Answer from the drawing. Dimensions are ordinates in mm from the lowest x, y and z of the part. A direction names the side the tool comes from. Coordinates: 2 decimals unless noted, no trailing zeros. Order: outer loops, then holes, each group sorted by start corner. A loop starts at its lowest first (then second) coordinate and runs counter-clockwise, first axis right, second up. Notation, with made-up numbers: (-11.5, 40.5) - (14.5, 40.5) arc R11 ccw to (14.5, 46.5) - close; hole circle Ø5 at (3, 69). An arc over 180 degrees is marked (long way). Answer as a JSON object with one key per item and string values. Group by question number.
1) Section C-C (y = 21) is taken. Give the vertices of the cut face in (x, z).
2) Section B-B (z = 1.95) is taken. Give the vertices of the cut face in (x, y).
3) Each of these flat-tipped pins is pushed along its axis until it touches: P1, Ø1, axis at x = 1, y = 21.5, coming from the -Z side; P2, Ø0.8, axis at x = 2.5, z = 3, coming from the +Y side. Where does it stop, or does it pass through?
4) The mould has two halves that part along X. Classify the marked faces 1, 2 and 3: released by +X, released by -X, zero draft, split by the parting line, or undercut.
5) Find the intervals of material crossed by line 1 along Z through (x, y) = (2.7, 9.5); line 2 along Y through (x, z) = (1.35, 4.45); line 3 along Y through (x, z) = (3.1, 2.4), in increasing order.
6) A tool of negligible diameter and unlimited length cuts with its end or side. For the marked faces 4 and 5, from which of +Z, -Z, +X, -X, +Y, -Y can it reach the whole face along a straight path? Write none if from no direction.
7) Section D-D (x = 0.5) is taken. Give the vertices of the cut face in (y, z).
8) Section A-A (x = 2.75) is taken. Give the vertices of the cut face in (y, z).
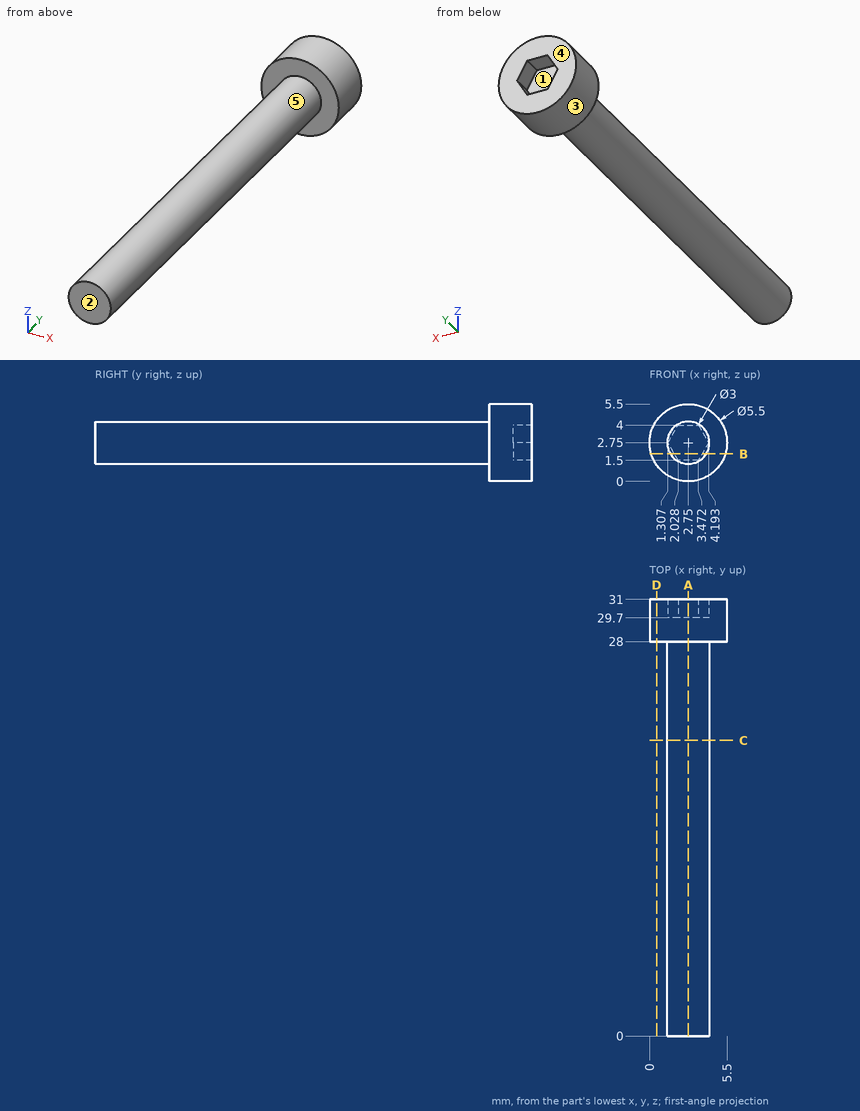
Report:
{
 "1": {"outline": "circle Ø3 at (2.75, 2.75)"},
 "2": {"outline": "(0.12, 28) - (1.48, 28) - (1.48, 0) - (4.02, 0) - (4.02, 28) - (5.38, 28) - (5.38, 31) - (3.73, 31) - (3.73, 29.7) - (1.77, 29.7) - (1.77, 31) - (0.12, 31) - close"},
 "3": {"P1": "stops at z = 1.92", "P2": "stops at y = 29.7"},
 "4": {"face 1": "undercut", "face 2": "zero draft", "face 3": "split by the parting line"},
 "5": {"line 1": "z = 1.25 to 4.25", "line 2": "y = 28 to 31", "line 3": "y = 0 to 29.7"},
 "6": {"face 4": "+Z, -Z, +X, -X, +Y", "face 5": "-Y"},
 "7": {"outline": "(28, 1.17) - (31, 1.17) - (31, 4.33) - (28, 4.33) - close"},
 "8": {"outline": "(0, 1.25) - (28, 1.25) - (28, 0) - (31, 0) - (31, 1.5) - (29.7, 1.5) - (29.7, 4) - (31, 4) - (31, 5.5) - (28, 5.5) - (28, 4.25) - (0, 4.25) - close"}
}
